The model under review builds one solid part; all positions refer to its coordinate system, in mm. Face numbers are marked on the shaded views. A direction names the side the tool comes from. Coordinates: 2 decimals unless noted, no trailing zeros. Order: outer loops, then holes, each group sorted by start corner. A loop starts at its lowest first (then second) coordinate and runs counter-clockwise, first axis right, second up.
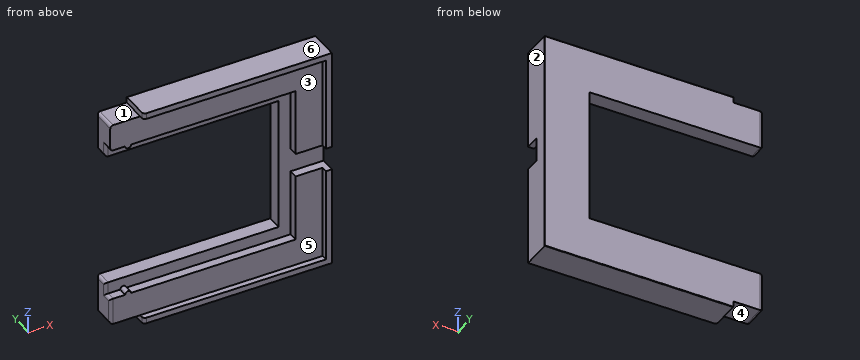
from build123d import *

# Parameters (mm, degrees)
PAD002_DEPTH       = 17.75
PAD002_DEPTH_BACK  = 17.75
POLARPATTERN_COUNT = 2
POLARPATTERN_ANGLE = 270
FILLET_R           = 0.5
PAD004_DEPTH       = 1.5
PAD005_DEPTH       = 5
FILLET005_R        = 0.1
FILLET006_R        = 0.5
FILLET007_R        = 0.5
SKETCH009_W        = 2.5
SKETCH009_H        = 4
POCKET001_DEPTH    = 36.501


with BuildPart() as part:
    # Sketch003 → Pad002 (new body, two sides)
    with BuildSketch(Plane.YZ) as pad002_sk:
        Polygon((0, -17.75), (4, -17.75), (4, -11.25), (1.5, -11.25), (1.5, -13.25), (0, -13.25), align=None)
    pad002 = extrude(amount=PAD002_DEPTH) + extrude(pad002_sk.sketch, amount=-PAD002_DEPTH_BACK)

    # PolarPattern: Pad002 ×2 about axis
    polarpattern_axis = Axis((0, 0, 0), (0, 1, 0))
    for i in range(1, POLARPATTERN_COUNT):
        add(pad002.rotate(polarpattern_axis, i * POLARPATTERN_ANGLE / (POLARPATTERN_COUNT - 1)))

    # Mirrored: Pad002 across Sketch003 H_Axis
    add(pad002.mirror(Plane.XY))

    # Fillet
    fillet_edges = [part.edges().sort_by_distance(p)[0] for p in [
        (-17.75, 4, 14.5),
        (-17.75, 2.75, 11.25),
        (-17.75, 0.75, 13.25),
        (-17.75, 1.5, 12.25),
        (-17.75, 2, 17.75),
    ]]
    fillet(fillet_edges, radius=FILLET_R)

    # Sketch007 → Pad004 (join)
    with BuildSketch(Plane(origin=(0, 1.5, 0), x_dir=(0, 0, -1), z_dir=(0, -1, 0))):
        with BuildLine():
            ThreePointArc((-13.25, -15.25), (-12.75, -14.75), (-13.25, -14.25))
            Line((-13.25, -14.25), (-13.25, -15.25))
        make_face()
    pad004 = extrude(amount=PAD004_DEPTH)

    # Sketch008 (on Face25 of Pad004) → Pad005 (join)
    with BuildSketch(Plane.ZX.offset(4)):
        Polygon((-18.75, 18.75), (18.75, 18.75), (18.75, -12.75), (17.75, -12.75), (17.75, 17.75), (-17.75, 17.75), (-17.75, -12.75), (-18.75, -12.75), align=None)
    extrude(amount=-PAD005_DEPTH)

    # Fillet005
    fillet005_edges = [part.edges().sort_by_distance(p)[0] for p in [
        (18.75, 4, 0),
        (3, 4, -18.75),
        (3, 4, 18.75),
    ]]
    fillet(fillet005_edges, radius=FILLET005_R)

    # Fillet006
    fillet006_edges = [part.edges().sort_by_distance(p)[0] for p in [
        (-17.75, 2.75, -11.25),
        (-17.75, 1.5, -12.25),
        (-17.75, 0, -15.5),
        (-17.75, 0.75, -13.25),
        (-17.75, 4, -14.5),
        (-17.75, 2, -17.75),
    ]]
    fillet(fillet006_edges, radius=FILLET006_R)

    # Fillet007
    fillet007_edges = [part.edges().sort_by_distance(p)[0] for p in [
        (-12.75, -1, 18.25),
        (-12.75, -1, -18.25),
    ]]
    fillet(fillet007_edges, radius=FILLET007_R)

    # Mirrored001: Pad004 across Sketch007 V_Axis
    add(pad004.mirror(Plane(origin=(0, 1.5, 0), x_dir=(0, -1, 0), z_dir=(0, 0, -1))))

    # Sketch009 (on Face9 of Mirrored001) → Pocket001 (cut, through all)
    with BuildSketch(Plane.YZ.offset(18.75)):
        with Locations((0.25, 0)):
            Rectangle(SKETCH009_W, SKETCH009_H)
    extrude(amount=-POCKET001_DEPTH, mode=Mode.SUBTRACT)


with BuildPart() as part_1:
    # Body001 placement: moved
    add(part.part.moved(Location((0, 0.3, 0))))


solid = part_1.part
(1) Wall thickness on line 1 (Z direction, x = 10, y = 0.75); line 2 (Z direction, x = -1, y = 3.3); line 3 (Y direction, x = 12, z = -3.5): over which ranges is each line inside the solid? List them lowest first.
(2) Consider section C-C (z = -8). Give the boundary of the cut face in (x, y).
(3) Tool access review of the marked faces 1, 2 and 3: name each direction out of +Z, -Z, +X, -X, +Y, -Y from which nothing blocks a thin tool from reaching the whole face with its end or side.
(4) Consider section D-D (x = -14.75). Give the boundary of the cut face in (y, z), then the cut area to 3 significant figures.
(5) The part is to be moulded in two halves that separate along Z. For the marked faces 4, 5 and 6, say which applies: +Z half, -Z half, draft (parallel to the pull), parting line (faces both ways), or undercut.
(6) Consider section A-A (x = -2). Give the boundary of the cut face in (y, z).
(7) Insertion check: pin 1 Ø17.5 at (x, z) = (4, -6.5) entering from -Y; pin 2 Ø12.5 at (x, z) = (-8, 6) entering from -Y; pin 3 Ø0.8 at (x, y) = (-16.5, 1) entering from -Z. Each pin has a flat end and moves straight along its axis. Give the tip position at first contact, or say it passes through.
(8) Consider section B-B (y = 3.3). Give the boundary of the cut face in (x, z).
Findings:
1. line 1: z = -18.75 to -13.25, 13.25 to 18.75
1. line 2: z = -18.75 to -11.25, 11.25 to 18.75
1. line 3: y = 1.8 to 4.3
2. outline: (11.25, 1.8) - (13.25, 1.8) - (13.25, 0.3) - (17.75, 0.3) - (17.75, -0.7) - (18.75, -0.7) - (18.75, 4.2) arc R0.1 ccw to (18.65, 4.3) - (11.25, 4.3) - close
3. face 1: +Z, -X, +Y, -Y
3. face 2: +Z, -Z, +X, +Y, -Y
3. face 3: -X, -Y
4. outline: (0.3, -17.75) - (4.3, -17.75) - (4.3, -11.25) - (1.8, -11.25) - (1.8, -12.75) - (0.3, -12.75) - close; (0.3, 12.75) - (1.8, 12.75) - (1.8, 11.25) - (4.3, 11.25) - (4.3, 17.75) - (0.3, 17.75) - close
4. area: 47.5 mm2
5. face 4: -Z half
5. face 5: undercut
5. face 6: +Z half
6. outline: (-0.7, -18.75) - (4.2, -18.75) arc R0.1 ccw to (4.3, -18.65) - (4.3, -11.25) - (1.8, -11.25) - (1.8, -13.25) - (0.3, -13.25) - (0.3, -17.75) - (-0.7, -17.75) - close; (-0.7, 17.75) - (0.3, 17.75) - (0.3, 13.25) - (1.8, 13.25) - (1.8, 11.25) - (4.3, 11.25) - (4.3, 18.65) arc R0.1 ccw to (4.2, 18.75) - (-0.7, 18.75) - close
7. pin 1: stops at y = 0.3
7. pin 2: stops at y = 1.8
7. pin 3: stops at z = -17.75
8. outline: (-17.75, -17.25) arc R0.5 ccw to (-17.25, -17.75) - (-12.75, -17.75) - (-12.75, -18.75) - (18.75, -18.75) - (18.75, 18.75) - (-12.75, 18.75) - (-12.75, 17.75) - (-17.25, 17.75) arc R0.5 ccw to (-17.75, 17.25) - (-17.75, 11.75) arc R0.5 ccw to (-17.25, 11.25) - (11.25, 11.25) - (11.25, -11.25) - (-17.25, -11.25) arc R0.5 ccw to (-17.75, -11.75) - close
